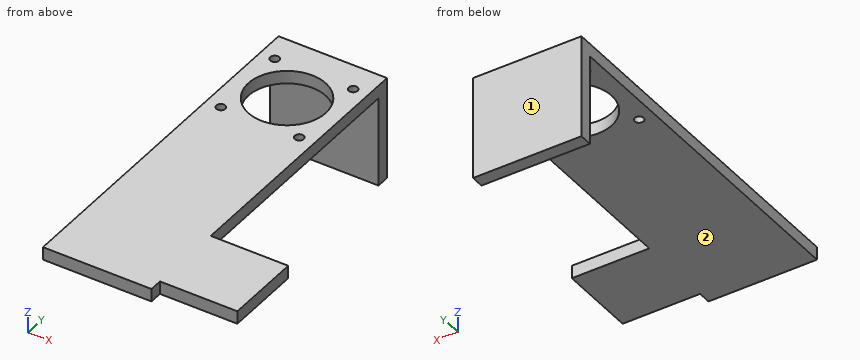
from build123d import *

# Parameters (mm, degrees)
SKETCH1_W                = 30
SKETCH1_H                = 30
SKETCH1_R                = 1.75
SKETCH1_R_2              = 15
BOSS_EXTRUDE1_DEPTH      = 5
SKETCH2_W                = 42
SKETCH2_H                = 5
BOSS_EXTRUDE3_DEPTH      = 35
BOSS_EXTRUDE3_DEPTH_BACK = 5


with BuildPart() as part:
    # Sketch1 → Boss-Extrude1 (new body)
    with BuildSketch(Plane.XY):
        with Locations((36, -92)):
            Rectangle(SKETCH1_W, SKETCH1_H)
        Polygon((-21, -22), (-21, -112), (21, -112), (21, -22), (21, 22), (-21, 22), align=None)
        with Locations((-15.190466427, 15.913821971)):
            Circle(SKETCH1_R, mode=Mode.SUBTRACT)
        with Locations((-15.190466427, -15.913821971)):
            Circle(SKETCH1_R, mode=Mode.SUBTRACT)
        with Locations((15.190466427, -15.913821971)):
            Circle(SKETCH1_R, mode=Mode.SUBTRACT)
        with Locations((15.190466427, 15.913821971)):
            Circle(SKETCH1_R, mode=Mode.SUBTRACT)
        Circle(SKETCH1_R_2, mode=Mode.SUBTRACT)
    extrude(amount=BOSS_EXTRUDE1_DEPTH)

    # Sketch2 → Boss-Extrude3 (add, two sides)
    with BuildSketch(Plane(origin=(0, 0, 0), x_dir=(-1, 0, 0), z_dir=(0, 0, -1))) as boss_extrude3_sk:
        with Locations((0, 24.5)):
            Rectangle(SKETCH2_W, SKETCH2_H)
    extrude(amount=BOSS_EXTRUDE3_DEPTH)
    extrude(boss_extrude3_sk.sketch, amount=-BOSS_EXTRUDE3_DEPTH_BACK)


solid = part.part
Geometry: final body of the model. Coordinates: model frame, mm. Face numbers are marked on the shaded views. A direction names the side the tool comes from. Give positions to 0.01 mm unless a question says otherwise; leave off trailing zeros. Write each loop counter-clockwise with the first axis right and the second up, starting at its lowest first coordinate (ties: lowest second). Pieces come first, ordered by that corner, then holes. Notation, with made-up numbers: (26, -25) -> (30, -25) arc R10 ccw to (30, -6) -> close; hole circle Ø8 at (24, 41.25). An arc over 180 degrees is marked (long way). Answer as a JSON object with one key per item and string values.
1. Contact query for flat-ended pins moving along their axis: pin 1 (5.5 mm diameter, centred on x = 43, z = 2, fed in from -Y); pin 2 (4 mm diameter, centred on x = -15.19, y = 15.91, fed in from -Z); pin 3 (24 mm diameter, centred on x = 0, y = 0, fed in from +Z); pin 4 (4 mm diameter, centred on x = 41.5, z = 2.5, fed in from +Y). Output: stop coordinate, or through.
Ans:
{"pin 1": "stops at y = -107", "pin 2": "stops at z = 0", "pin 3": "passes through", "pin 4": "stops at y = -77"}
2. Access query for the marked faces 1 and 2. Directions: +Z, -Z, +X, -X, +Y, -Y. A direction counts if a zero-diameter tool reaches every point of the face in a straight line with its end or side. Return the directions, or none.
Ans:
{"face 1": "+Z, -Z, +X, -X, +Y", "face 2": "-Z, +X, -X, -Y"}
3. Cut plane B-B on y = 0. Output: boundary loops of the cut face in (x, z), and give its area (3 significant figures).
Ans:
{"outline": "(-21, 0) -> (-15, 0) -> (-15, 5) -> (-21, 5) -> close; (15, 0) -> (21, 0) -> (21, 5) -> (15, 5) -> close", "area": "60.0 mm^2"}
4. Cut plane D-D on y = -99. Output: boundary loops of the cut face in (x, z).
Ans:
{"outline": "(-21, 0) -> (51, 0) -> (51, 5) -> (-21, 5) -> close"}
5. Ray query, probe 1 along Y at (x, z) = (-10.5, -27.5); probe 2 along Y at (x, z) = (0, 1); probe 3 along Z at (x, y) = (17, -49). Return the intervals inside material, ascending. Write a range as from..to.
Ans:
{"probe 1": "y = 22..27", "probe 2": "y = -112..-15, 15..27", "probe 3": "z = 0..5"}
6. Cut plane C-C on z = -16. Output: boundary loops of the cut face in (x, y), and give its area (3 significant figures).
Ans:
{"outline": "(-21, 22) -> (21, 22) -> (21, 27) -> (-21, 27) -> close", "area": "210 mm^2"}
7. Cut plane A-A on x = 0. Output: boundary loops of the cut face in (y, z), and give its area (3 significant figures).
Ans:
{"outline": "(-112, 0) -> (-15, 0) -> (-15, 5) -> (-112, 5) -> close; (15, 0) -> (22, 0) -> (22, -35) -> (27, -35) -> (27, 5) -> (15, 5) -> close", "area": "720 mm^2"}
